```python
from build123d import *

# Parameters (mm, degrees)
EXTRUDE_1_DEPTH     = 20
CUT_EXTRUDE_START   = 3
CUT_EXTRUDE_1_DEPTH = 2
EXTRUDE_2_DEPTH     = 3
SKETCH_115_R        = 2
SKETCH_115_R_2      = 1.5
CUT_EXTRUDE_2_DEPTH = 279.143495269
FILLET_1_R          = 5
SKETCH_116_R        = 2
CUT_EXTRUDE_3_DEPTH = 279.143495269


with BuildPart() as part:
    # 草图1 → 凸台-拉伸1 (new body)
    with BuildSketch(Plane(origin=(0, 0, 0), x_dir=(-1, 0, 0), z_dir=(0, 0, 1))):
        Polygon((74.438153655, 158.80166336), (74.438153655, 150.81385389), (66.84370456, 145.696765598), (60.754110218, 149.581447702), (55.174801085, 164.459776844), (47.261962171, 267.008923523), (57.886031057, 267.008923523), (68.150536307, 171.985087167), align=None)
    extrude(amount=EXTRUDE_1_DEPTH)

    # 草图113 → 切除-拉伸1 (cut)
    with BuildSketch(Plane(origin=(0, 0, 10), x_dir=(-1, 0, 0), z_dir=(0, 0, -1)).offset(CUT_EXTRUDE_START)):
        Polygon((55.174801085, -164.459776844), (47.261962171, -267.008923523), (57.886031057, -267.008923523), (68.150536307, -171.985087167), (74.438153655, -158.80166336), (74.438153655, -150.81385389), (66.84370456, -145.696765598), (60.754110218, -149.581447702), align=None)
        Polygon((56.653989783, -164.787273226), (48.882163106, -265.508923523), (56.539335626, -265.508923523), (66.686650777, -171.56997655), (72.938153655, -158.462274967), (72.938153655, -151.61189122), (66.821209313, -147.490335609), (61.982843766, -150.576832179), align=None, mode=Mode.SUBTRACT)
    cut_extrude_1 = extrude(amount=CUT_EXTRUDE_1_DEPTH, mode=Mode.SUBTRACT)

    # 镜向1: 切除-拉伸1 across plane
    add(cut_extrude_1.mirror(Plane(origin=(0, 0, 10), x_dir=(1, 0, 0), z_dir=(0, 0, -1))), mode=Mode.SUBTRACT)

    # 草图114 → 凸台-拉伸2 (add)
    with BuildSketch(Plane(origin=(0, 0, 0), x_dir=(-1, 0, 0), z_dir=(0, 0, -1))):
        with BuildLine():
            Line((58.025627707, -173.935710741), (57.419339245, -181.793113798))
            ThreePointArc((57.419339245, -181.793113798), (57.684559456, -182.273815488), (58.231058467, -182.221330198))
            Line((58.231058467, -182.221330198), (62.923737604, -178.450317813))
            ThreePointArc((62.923737604, -178.450317813), (63.109801357, -178.087671778), (62.964089914, -177.707014396))
            Line((62.964089914, -177.707014396), (58.877699239, -173.620623723))
            ThreePointArc((58.877699239, -173.620623723), (58.350728284, -173.505214058), (58.025627707, -173.935710741))
        make_face()
        with BuildLine():
            Line((60.934012548, -197.454954781), (56.971204979, -194.518647305))
            ThreePointArc((56.971204979, -194.518647305), (56.448628412, -194.473820011), (56.173532656, -194.920382527))
            Line((56.173532656, -194.920382527), (56.173532659, -203.204850558))
            ThreePointArc((56.173532659, -203.204850558), (56.516796592, -203.679649258), (57.07526788, -203.50252288))
            Line((57.07526788, -203.50252288), (61.038075447, -198.154362325))
            ThreePointArc((61.038075447, -198.154362325), (61.130896043, -197.783106421), (60.934012548, -197.454954781))
        make_face()
        with BuildLine():
            Line((57.978905554, -188.563420266), (61.66084791, -192.808841031))
            ThreePointArc((61.66084791, -192.808841031), (62.213413835, -192.949681307), (62.538578919, -192.481244809))
            Line((62.538578919, -192.481244809), (62.538578917, -185.277034446))
            ThreePointArc((62.538578917, -185.277034446), (62.25468012, -184.826146133), (61.725377837, -184.887284419))
            Line((61.725377837, -184.887284419), (58.043435482, -187.846074018))
            ThreePointArc((58.043435482, -187.846074018), (57.858647408, -188.191026703), (57.978905554, -188.563420266))
        make_face()
        with BuildLine():
            Line((59.442872047, -206.313835661), (56.081759275, -208.539915803))
            ThreePointArc((56.081759275, -208.539915803), (55.862445165, -208.889140713), (55.980118188, -209.284374538))
            Line((55.980118188, -209.284374538), (59.341230961, -213.159866488))
            ThreePointArc((59.341230961, -213.159866488), (59.893796886, -213.300706764), (60.218961971, -212.832270266))
            Line((60.218961971, -212.832270266), (60.218961969, -206.730698174))
            ThreePointArc((60.218961969, -206.730698174), (59.955557657, -206.290218344), (59.442872047, -206.313835661))
        make_face()
        with BuildLine():
            Line((59.180756665, -219.162865233), (55.202116295, -215.184224865))
            ThreePointArc((55.202116295, -215.184224865), (54.657221188, -215.07583849), (54.348562904, -215.537778256))
            Line((54.348562904, -215.537778256), (54.348562906, -222.366147911))
            ThreePointArc((54.348562906, -222.366147911), (54.620062064, -222.810880826), (55.139712367, -222.772635293))
            Line((55.139712367, -222.772635293), (59.118352735, -219.922906006))
            ThreePointArc((59.118352735, -219.922906006), (59.325526398, -219.557333957), (59.180756665, -219.162865233))
        make_face()
        with BuildLine():
            Line((57.496934877, -227.057752455), (54.36647935, -229.299963354))
            ThreePointArc((54.36647935, -229.299963354), (54.158945852, -229.670183565), (54.310729697, -230.066535456))
            Line((54.310729697, -230.066535456), (57.441185226, -233.082359755))
            ThreePointArc((57.441185226, -233.082359755), (57.983724881, -233.182410645), (58.288084339, -232.722275036))
            Line((58.288084339, -232.722275036), (58.288084338, -227.464239836))
            ThreePointArc((58.288084338, -227.464239836), (58.01658518, -227.019506922), (57.496934877, -227.057752455))
        make_face()
    extrude_2 = extrude(amount=EXTRUDE_2_DEPTH)

    # 镜向2: 凸台-拉伸2 across plane
    add(extrude_2.mirror(Plane(origin=(0, 0, 10), x_dir=(1, 0, 0), z_dir=(0, 0, -1))))

    # 草图115 → 切除-拉伸2 (cut, through all)
    with BuildSketch(Plane(origin=(0, 0, 0), x_dir=(-1, 0, 0), z_dir=(0, 0, -1))):
        with Locations((64.915803172, -164.949805196)):
            Circle(SKETCH_115_R)
        with Locations((67.132054217, -155.644675734)):
            Circle(SKETCH_115_R)
        with Locations((54.86719071, -241.489374019)):
            Circle(SKETCH_115_R_2)
    extrude(amount=-CUT_EXTRUDE_2_DEPTH, mode=Mode.SUBTRACT)

    # 圆角1
    fillet_1_edges = [part.edges().sort_by_distance(p)[0] for p in [
        (-74.438153655, -150.81385389, 17.5),
        (-66.84370456, -145.696765598, 17.5),
        (-74.438153655, -150.81385389, 2.5),
        (-66.84370456, -145.696765598, 2.5),
        (-66.84370456, -145.696765598, 10),
        (-74.438153655, -150.81385389, 10),
    ]]
    fillet(fillet_1_edges, radius=FILLET_1_R)

    # 草图116 → 切除-拉伸3 (cut, through all)
    with BuildSketch(Plane(origin=(0, 0, 0), x_dir=(-1, 0, 0), z_dir=(0, 0, -1))):
        with Locations((53.184824598, -261.558408948)):
            Circle(SKETCH_116_R)
    extrude(amount=-CUT_EXTRUDE_3_DEPTH, mode=Mode.SUBTRACT)


solid = part.part
```
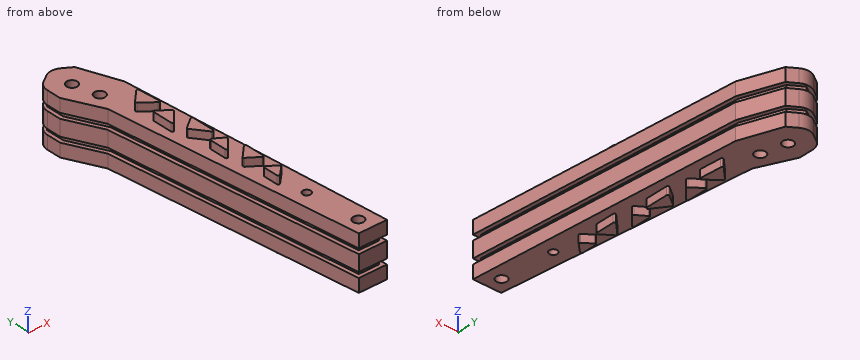
Could you check a few things on this model? Use its own coordinates, in mm. Give positions to 0.01 mm unless a question says otherwise; leave off trailing zeros. Order: outer loops, then holes, each group sorted by start corner. A loop starts at its lowest first (then second) coordinate and runs counter-clockwise, first axis right, second up.
Q1. Suppose I cut it at C-C, the plane y = -235. Write out the boundary of the cut face in (x, z).
Q2. Suppose I cut it at A-A, the plane z = 11.25. Write out the boundary of the cut face in (x, y).
Q3. If I drill on line 1 along Z through (x, y) = (-52.5, -201); line 2 along Z through (x, y) = (-65, -179); line 3 along X through (y, z) = (-158.5, 18.5), over which ranges is the centre line in solid material (lowest first)?
Q4. Suppose I cut it at B-B, the plane y = -258. Write out the boundary of the cut face in (x, z), and give its area (3 significant figures).
Q5. I'm going to push flat-ended pins straight in: P1, Ø1.6, axis at y = -155.5, z = 14, coming from the -X side; P2, Ø0.6, axis at x = -53, z = 14.5, coming from the -Y side; P3, Ø6, axis at x = -63.5, y = -212.5, coming from the -Z side. Where does each tip first touch, or does it pass through?
Solution:
1. outline: (-61.34, 0) - (-49.73, 0) - (-49.73, 5) - (-51.24, 5) - (-51.24, 7) - (-49.73, 7) - (-49.73, 13) - (-51.24, 13) - (-51.24, 15) - (-49.73, 15) - (-49.73, 20) - (-61.34, 20) - (-61.34, 15) - (-59.83, 15) - (-59.83, 13) - (-61.34, 13) - (-61.34, 7) - (-59.83, 7) - (-59.83, 5) - (-61.34, 5) - close
2. outline: (-74.44, -158.8) - (-68.15, -171.99) - (-57.89, -267.01) - (-47.26, -267.01) - (-55.17, -164.46) - (-60.75, -149.58) - (-64.08, -147.46) arc R5 ccw to (-69.56, -147.53) - (-72.23, -149.33) arc R5 ccw to (-74.44, -153.47) - close; hole circle Ø4 at (-67.13, -155.64); hole circle Ø4 at (-64.92, -164.95); hole circle Ø3 at (-54.87, -241.49); hole circle Ø4 at (-53.18, -261.56)
3. line 1: z = 0 to 5, 7 to 13, 15 to 20
3. line 2: z = 0 to 20
3. line 3: x = -74.44 to -57.41
4. outline: (-58.86, 0) - (-47.96, 0) - (-47.96, 5) - (-49.46, 5) - (-49.46, 7) - (-47.96, 7) - (-47.96, 13) - (-49.46, 13) - (-49.46, 15) - (-47.96, 15) - (-47.96, 20) - (-58.86, 20) - (-58.86, 15) - (-57.35, 15) - (-57.35, 13) - (-58.86, 13) - (-58.86, 7) - (-57.35, 7) - (-57.35, 5) - (-58.86, 5) - close
4. area: 206 mm2
5. P1: stops at x = -72.94
5. P2: stops at y = -265.51
5. P3: stops at z = 0
